The model under review builds one solid part; all positions refer to its coordinate system, in mm. A direction names the side the tool comes from. Round coordinates to 2 decimals unless told otherwise and drop trailing zeros. Order: outer loops, then holes, each group sorted by start corner. A loop starts at its lowest first (then second) coordinate and runs counter-clockwise, first axis right, second up. Notation, with made-up numbers: (38, 85.25) -> (68, 85.25) arc R15 cw to (68, 113.25) -> close; hole circle Ø5 at (-32.5, 84). An arc over 180 degrees is marked (long way). Use a Markdown table: item, result. Add a question column.
```python
from build123d import *
from OCP.BRepFilletAPI import BRepFilletAPI_MakeChamfer

# Parameters (mm, degrees)
SKETCH1_W           = 20
SKETCH1_H           = 6
SKETCH1_R           = 1.25
BOSS_EXTRUDE1_DEPTH = 3
SKETCH2_W           = 13
SKETCH2_H           = 6
CUT_EXTRUDE1_DEPTH  = 1.25
CHAMFER1_SIZE       = 2
SKETCH3_R           = 1.75
SKETCH3_R_2         = 1.25
BOSS_EXTRUDE2_DEPTH = 7.5
CHAMFER2_SIZE       = 0.525155654
CHAMFER2_SIZE_2     = 0.75
CHAMFER3_SIZE       = 1.25
CHAMFER3_SIZE_2     = 0.875259423


# Some blends are built 0.0001 mm under size
with BuildPart() as part:
    # Sketch1 → Boss-Extrude1 (new body)
    with BuildSketch(Plane(origin=(0, 0, 0), x_dir=(1, 0, 0), z_dir=(0, 1, 0))):
        Rectangle(SKETCH1_W, SKETCH1_H)
        with Locations(Location((-8.25, 0, 0), (0, 0, 270))):
            Circle(SKETCH1_R, mode=Mode.SUBTRACT)
        with Locations(Location((8.25, 0, 0), (0, 0, 90))):
            Circle(SKETCH1_R, mode=Mode.SUBTRACT)
    extrude(amount=BOSS_EXTRUDE1_DEPTH)

    # Sketch2 → Cut-Extrude1 (cut)
    with BuildSketch(Plane(origin=(0, 3, 0), x_dir=(1, 0, 0), z_dir=(0, 1, 0))):
        Rectangle(SKETCH2_W, SKETCH2_H)
    extrude(amount=-CUT_EXTRUDE1_DEPTH, mode=Mode.SUBTRACT)

    # Chamfer1
    chamfer1_edges = [part.edges().sort_by_distance(p)[0] for p in [
        (10, 1.5, 3),
        (-10, 1.5, 3),
        (-10, 1.5, -3),
        (10, 1.5, -3),
    ]]
    chamfer(chamfer1_edges, length=CHAMFER1_SIZE)

    # Sketch3 → Boss-Extrude2 (add)
    with BuildSketch(Plane(origin=(0, 3, 0), x_dir=(1, 0, 0), z_dir=(0, 1, 0))):
        with Locations(Location((-8.25, 0, 0), (0, 0, 180))):
            Circle(SKETCH3_R)
        with Locations(Location((-8.25, 0, 0), (0, 0, 270))):
            Circle(SKETCH3_R_2, mode=Mode.SUBTRACT)
    boss_extrude2 = extrude(amount=BOSS_EXTRUDE2_DEPTH)

    # Mirror1: Boss-Extrude2 across plane
    add(boss_extrude2.mirror(Plane(origin=(0, 0, 0), x_dir=(0, 0, 1), z_dir=(1, 0, 0))))

    # Chamfer2
    # the kernel refuses this chamfer: 0.75, 0.525155654 mm, written as the material it takes off along each edge
    with BuildSketch(Plane(origin=(-8.25, 0, 0), x_dir=(0, 0, 1), z_dir=(-1, 0, 0))) as chamfer2_piece_1:
        Polygon((1.25 + CHAMFER2_SIZE, 0), (1.25, CHAMFER2_SIZE_2), (1.25, 0), align=None)
    revolve(axis=Axis((-8.25, 0, 0), (0, 1, 0)), mode=Mode.SUBTRACT)
    with BuildSketch(Plane(origin=(8.25, 0, 0), x_dir=(0, 0, -1), z_dir=(1, 0, 0))) as chamfer2_piece_2:
        Polygon((1.25 + CHAMFER2_SIZE, 0), (1.25, CHAMFER2_SIZE_2), (1.25, 0), align=None)
    revolve(axis=Axis((8.25, 0, 0), (0, 1, 0)), mode=Mode.SUBTRACT)

    # Chamfer3
    chamfer3_edges_1 = [part.edges().sort_by_distance(p)[0] for p in [
        (6.5, 1.75, 0),
    ]]
    chamfer3_side_1 = [part.faces().sort_by_distance(p)[0] for p in [
        (6.5, 1.767505188, 0),
    ]]
    chamfer3_edges_2 = [part.edges().sort_by_distance(p)[0] for p in [
        (-6.5, 1.75, 0),
    ]]
    chamfer3_side_2 = [part.faces().sort_by_distance(p)[0] for p in [
        (-6.5, 1.767505188, 0),
    ]]
    chamfer3 = BRepFilletAPI_MakeChamfer(part.part.solid().wrapped)
    for e in chamfer3_edges_1:
        chamfer3.Add(CHAMFER3_SIZE - 0.0001, CHAMFER3_SIZE_2 - 0.0001, e.wrapped, chamfer3_side_1[0].wrapped)
    for e in chamfer3_edges_2:
        chamfer3.Add(CHAMFER3_SIZE - 0.0001, CHAMFER3_SIZE_2 - 0.0001, e.wrapped, chamfer3_side_2[0].wrapped)
    add(Compound.cast(chamfer3.Shape()), mode=Mode.REPLACE)  # a hair under: the kernel refuses the full size


solid = part.part
```
Q1. Add section A-A (x = 8.25). Write out the cut boundary in (y, z).
Q2. Add section D-D (x = 2.25). Write out the cut boundary in (y, z).
Q3. Add section B-B (y = 3.75). Write out the cut boundary in (x, z), then the cut area to 3 significant figures.
Q4. Mouldability with a two-part tool opening along Z and no side actions: class faces 1 (the flat face through (9, 1, -2)), 2 (the flat face through (-9.4, 10.5, -0.8)), 3 (the cylindrical face through (-9.919, 6.698, 0.526)) as pulls with the +Z half, pulls with the -Z half, needs draft (parallel to the pull), parting line crosses it, or undercut.
Q5. Add section C-C (z = 0.75). State how many separate pieces and enclosed holes the cut face has, then the cut area to 3 significant figures.
Q6. Insertion check: pin 1 (1.5 mm diameter, centred on x = -8.25, z = 0, fed in from +Y); pin 2 (3 mm diameter, centred on x = 0.5, z = -1, fed in from +Y); pin 3 (1 mm diameter, centred on x = -6.5, z = -2, fed in from +Y); pin 4 (1 mm diameter, centred on y = 4.5, z = -2, fed in from -X). Each pin has a flat end and moves straight along its axis. Give the tip position at first contact, or say it passes through.
Q7. Machinability: for faces 4 (the flat face through (-6.06, 2.37, 0.04)), 5 (the flat face through (-8, 3, -2)), 6 (the cylindrical face through (9.919, 6.698, 0.526)), which of the approach directions +Z, -Z, +X, -X, +Y, -Y give a long, thin tool a straight path to every point of the face, cutting with its end or side? Answer none if there is none.
Q8. Wall thickness on line 1 (Z direction, x = 8.25, y = 5.75); line 2 (X direction, y = 1.25, z = 0); line 3 (X direction, y = 4.75, z = 0.25): over which ranges is each line inside the solid? List them lowest first. Write a range as [from, to].
Report:
| question | item | result |
|---|---|---|
| 1 | outline | (0, -2.75) -> (3, -2.75) -> (3, -1.75) -> (10.5, -1.75) -> (10.5, -1.25) -> (0.75, -1.25) -> (0, -1.78) -> close; (0, 1.78) -> (0.75, 1.25) -> (10.5, 1.25) -> (10.5, 1.75) -> (3, 1.75) -> (3, 2.75) -> (0, 2.75) -> close |
| 2 | outline | (0, -3) -> (1.75, -3) -> (1.75, 3) -> (0, 3) -> close |
| 3 | outline | circle Ø3.5 at (-8.25, 0); circle Ø3.5 at (8.25, 0); hole circle Ø2.5 at (-8.25, 0); hole circle Ø2.5 at (8.25, 0) |
| 3 | area | 9.42 mm² |
| 4 | face 1 | pulls with the -Z half |
| 4 | face 2 | needs draft |
| 4 | face 3 | parting line crosses it |
| 5 | separate pieces | 3 |
| 5 | enclosed holes | 0 |
| 5 | area | 49.3 mm² |
| 6 | pin 1 | passes through |
| 6 | pin 2 | stops at y = 1.75 |
| 6 | pin 3 | stops at y = 3 |
| 6 | pin 4 | stops at x = -9.15 |
| 7 | face 4 | +Z, -Z, +Y |
| 7 | face 5 | -Z, +Y |
| 7 | face 6 | +Y |
| 8 | line 1 | z = [-1.75, -1.25], [1.25, 1.75] |
| 8 | line 2 | x = [-10, -9.5], [-7, 7], [9.5, 10] |
| 8 | line 3 | x = [-9.98, -9.47], [-7.03, -6.52], [6.52, 7.03], [9.47, 9.98] |
